Geometry: final body of the model. Coordinates: model frame, mm. Face numbers are marked on the shaded views. A direction names the side the tool comes from. Give positions to 0.01 mm unless a question says otherwise; leave off trailing zeros. Write each loop counter-clockwise with the first axis right and the second up, starting at its lowest first coordinate (ties: lowest second). Pieces come first, ordered by that corner, then holes. Notation, with made-up numbers: M -9,-22.75 L -4,-22.75 A18 cw -4,-14.75 Z; hole C 79.25,-7.75 d9. An arc over 180 degrees is marked long. Use one line per item in the form item = value. Start each with the question number.
Item 1: Access query for the marked faces 4, 5 and 6. Directions: +Z, -Z, +X, -X, +Y, -Y. A direction counts if a zero-diameter tool reaches every point of the face in a straight line with its end or side. Return the directions, or none.
Item 2: Section query A-A on z = 24. Return loops of the section in (x, y).
Item 3: Pull-direction query (Z, two-part tool) for the marked faces 1, 2 and 3; classes: released by +Z, released by -Z, zero draft, split by the parting line, or undercut.
Item 4: Material intervals for line 1 along Z through (x, y) = (30, -5.5); line 2 along X through (y, z) = (-4, 40.5); line 3 along X through (y, z) = (-1, 7), sorted ascending. Write a range as from..to.
Item 5: Section query D-D on z = 46. Return loops of the section in (x, y).
Item 6: Section query C-C on z = 55. Return loops of the section in (x, y).
Item 7: Contact query for flat-ended pins moving along their axis: P1, Ø9, axis at y = -4, z = 69.5, coming from the -X side; P2, Ø1, axis at x = 16, y = -5.5, coming from the -Z side; P3, Ø4, axis at y = -4.5, z = 7, coming from the -X side. Output: stop coordinate, or through.
Item 8: Section query B-B on x = 26.5. Return loops of the section in (y, z), then the cut area to 3 significant figures.
from build123d import *

# Parameters (mm, degrees)
F1_DEPTH = 15


with BuildPart() as f1:
    # F0 (on Front) → F1 (new body)
    with BuildSketch(Plane.XZ):
        Polygon((23.861149, 25.248436), (35.014816, 31.688008), (35.014816, 18.401567), (25.119459, 11.732958), (28.74309, 6.355957), (35.049491, 10.605923), (35.049491, 2.554659), (41.755129, 2.554659), (41.755129, 10.729081), (47.921799, 6.426754), (51.6238, 11.732958), (41.577444, 18.742041), (41.577444, 31.621186), (53.08384, 24.977965), (53.911346, 13.074031), (60.379781, 13.523686), (59.852403, 21.110173), (66.825002, 17.084541), (70.177821, 22.891793), (63.098564, 26.979004), (69.907824, 30.168334), (67.163517, 36.027463), (56.070295, 30.831605), (44.916629, 37.271177), (56.423024, 43.914398), (67.145887, 38.679072), (69.990691, 44.505729), (63.156912, 47.84225), (70.129511, 51.867882), (66.776692, 57.675134), (59.697435, 53.587923), (60.340024, 61.07958), (53.893716, 61.632505), (52.846851, 49.427564), (41.693184, 42.987992), (41.693184, 56.274433), (51.588541, 62.943042), (47.96491, 68.320043), (41.658509, 64.070077), (41.658509, 72.121341), (34.952871, 72.121341), (34.952871, 63.946919), (28.786201, 68.249246), (25.0842, 62.943042), (35.130556, 55.933959), (35.130556, 43.054814), (23.62416, 49.698035), (22.796654, 61.601969), (16.328219, 61.152314), (16.855597, 53.565827), (9.882998, 57.591459), (6.530179, 51.784207), (13.609436, 47.696996), (6.800176, 44.507666), (9.544483, 38.648537), (20.637705, 43.844395), (31.791371, 37.404823), (20.284976, 30.761602), (9.562113, 35.996928), (6.717309, 30.170271), (13.551088, 26.83375), (6.578489, 22.808118), (9.931308, 17.000866), (17.010565, 21.088077), (16.367976, 13.59642), (22.814284, 13.043495), align=None)
    extrude(amount=F1_DEPTH)


solid = f1.part
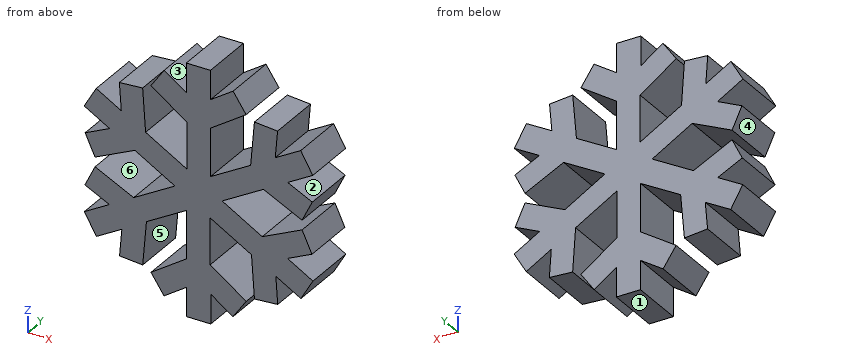
Answer sheet:
q1.face_4 = -X, +Y, -Y
q1.face_5 = -Z, +Y, -Y
q1.face_6 = +Y, -Y
q2.outline = M 8.64,-15 L 23.75,-15 L 23.75,0 L 8.64,0 Z; M 35.01,-15 L 41.58,-15 L 41.58,0 L 35.01,0 Z; M 53.15,-15 L 68.26,-15 L 68.26,0 L 53.15,0 Z
q3.face_1 = released by -Z
q3.face_2 = undercut
q3.face_3 = released by +Z
q4.line_1 = 7.2..15.02, 28.79..36.37, 38.44..46.02, 59.51..67.4
q4.line_2 = 8.68..13.5, 26.43..50.51, 63.42..68.03
q4.line_3 = 28.31..29.7, 35.05..41.76, 47.1..48.32
q5.outline = M 9.99,-15 L 30.03,-15 L 30.03,0 L 9.99,0 Z; M 35.13,-15 L 41.69,-15 L 41.69,0 L 35.13,0 Z; M 46.91,-15 L 66.93,-15 L 66.93,0 L 46.91,0 Z
q6.outline = M 8.39,-15 L 14.37,-15 L 14.37,0 L 8.39,0 Z; M 16.76,-15 L 23.26,-15 L 23.26,0 L 16.76,0 Z; M 35.13,-15 L 41.69,-15 L 41.69,0 L 35.13,0 Z; M 53.32,-15 L 59.82,-15 L 59.82,0 L 53.32,0 Z; M 62.14,-15 L 68.32,-15 L 68.32,0 L 62.14,0 Z
q7.P1 = 26.52
q7.P2 = 13.59
q7.P3 = 26.96
q8.outline = M -15,9.68 L 0,9.68 L 0,12.66 L -15,12.66 Z; M -15,26.77 L 0,26.77 L 0,34.35 L -15,34.35 Z; M -15,40.46 L 0,40.46 L 0,48.04 L -15,48.04 Z; M -15,61.96 L 0,61.96 L 0,64.97 L -15,64.97 Z
q8.area = 317 mm2
